```python
from build123d import *

# Parameters (mm, degrees)
F0_R     = 1.45
F1_DEPTH = 5


# Not quite as in the source:
# - ends of sketch curves that miss each other by under 0.0002 mm in the source are joined


with BuildPart() as f1:
    # F0 (on Top) → F1 (new body)
    with BuildSketch(Plane.XY):
        Polygon((-0.3545266845, 90.9670817697), (-29.9807621135, 108.0717967697), (-35.7307621135, 98.1125046262), (-37.3235262825, 82.9583658326), (-71.3455488748, 86.5342244993), (-72.5476262023, 75.0972227026), (-67.8389451324, 60.6053924919), (-100.3740420816, 50.0340986743), (-96.8203466463, 39.0969487369), (-86.6243940714, 27.7731962067), (-112.046951543, 4.8826226429), (-104.3519495698, -3.6635428501), (-90.4316983176, -9.8612380143), (-104.345925168, -41.1131032006), (-93.8401524051, -45.790574596), (-78.6025403784, -45.790574596), (-78.6025403784, -80), (-67.1025403784, -80), (-53.1822891262, -73.8023048358), (-39.2680622758, -105.0541700222), (-28.7622895129, -100.3766986268), (-18.5663369381, -89.0529460966), (6.8562205334, -111.9435196603), (14.5512225065, -103.3973541673), (19.2599035765, -88.9055239566), (51.7950005256, -99.4768177743), (55.3486959609, -88.5396678369), (53.7559317919, -73.3855290433), (87.7779543842, -69.8096703765), (86.5758770566, -58.3726685798), (78.9570710433, -45.1765094717), (108.583302492, -28.0717967697), (102.833302492, -18.1125046262), (90.5058154087, -9.1560609968), (110.6136111506, 18.5199455228), (101.3099157153, 25.2794759242), (86.4052820705, 28.4475536047), (93.5178215482, 61.9094209861), (82.2691241397, 64.3004054305), (67.364490495, 61.13232775), (60.2519510173, 94.5941951314), (49.0032536089, 92.203210687), (36.6757665257, 83.2467670575), (16.5679707838, 110.9227735772), (7.2642753485, 104.1632431758), align=None)
        with Locations((-73.1025403784, -73)):
            Circle(F0_R, mode=Mode.SUBTRACT)
        with Locations((-73.1025403784, -57)):
            Circle(F0_R, mode=Mode.SUBTRACT)
        with Locations((-37.0907187603, -96.4223002818)):
            Circle(F0_R, mode=Mode.SUBTRACT)
        with Locations((-6.5558921176, -92.4662191739)):
            Circle(F0_R, mode=Mode.SUBTRACT)
        with Locations((-43.5985050495, -81.8055729595)):
            Circle(F0_R, mode=Mode.SUBTRACT)
        with Locations((-96.4742686494, -36.9553365341)):
            Circle(F0_R, mode=Mode.SUBTRACT)
        with Locations((-89.9664823602, -22.3386092118)):
            Circle(F0_R, mode=Mode.SUBTRACT)
        with Locations((5.33442509, -103.1723088757)):
            Circle(F0_R, mode=Mode.SUBTRACT)
        with Locations((31.6202941199, -87.138616064)):
            Circle(F0_R, mode=Mode.SUBTRACT)
        with Locations((46.8371983806, -92.082887974)):
            Circle(F0_R, mode=Mode.SUBTRACT)
        with Locations((64.3290442427, -66.7439546071)):
            Circle(F0_R, mode=Mode.SUBTRACT)
        with Locations((80.2413945686, -65.0714991949)):
            Circle(F0_R, mode=Mode.SUBTRACT)
        with Locations((85.9147182049, -34.8086570489)):
            Circle(F0_R, mode=Mode.SUBTRACT)
        with Locations((99.7711246655, -26.8086570489)):
            Circle(F0_R, mode=Mode.SUBTRACT)
        with Locations((-103.1647194297, 5.4792403473)):
            Circle(F0_R, mode=Mode.SUBTRACT)
        with Locations((-91.274402222, 16.185330049)):
            Circle(F0_R, mode=Mode.SUBTRACT)
        with Locations((-92.0170529985, 46.9664067953)):
            Circle(F0_R, mode=Mode.SUBTRACT)
        with Locations((-76.8001487377, 51.9106787053)):
            Circle(F0_R, mode=Mode.SUBTRACT)
        with Locations((-64.9588021552, 80.3326548319)):
            Circle(F0_R, mode=Mode.SUBTRACT)
        with Locations((-49.0464518293, 78.6601994197)):
            Circle(F0_R, mode=Mode.SUBTRACT)
        with Locations((-12.8121778265, 91.8086570489)):
            Circle(F0_R, mode=Mode.SUBTRACT)
        with Locations((-26.668584287, 99.8086570489)):
            Circle(F0_R, mode=Mode.SUBTRACT)
        with Locations((92.6449568788, 3.1453735398)):
            Circle(F0_R, mode=Mode.SUBTRACT)
        with Locations((102.0495209155, 16.0896454498)):
            Circle(F0_R, mode=Mode.SUBTRACT)
        with Locations((83.3560408553, 40.5555404687)):
            Circle(F0_R, mode=Mode.SUBTRACT)
        with Locations((25.6374381175, 89.0825638189)):
            Circle(F0_R, mode=Mode.SUBTRACT)
        with Locations((16.2328740808, 102.0268357289)):
            Circle(F0_R, mode=Mode.SUBTRACT)
        with Locations((59.6541081021, 70.953286015)):
            Circle(F0_R, mode=Mode.SUBTRACT)
        with Locations((86.6826279084, 56.2059020804)):
            Circle(F0_R, mode=Mode.SUBTRACT)
        with Locations((56.327521049, 86.6036476267)):
            Circle(F0_R, mode=Mode.SUBTRACT)
    extrude(amount=F1_DEPTH)


solid = f1.part
```
Input: part model. Units: mm. Frame: model coordinates. A direction names the side the tool comes from. Give positions to 0.01 mm unless a question says otherwise; leave off trailing zeros. Order: outer loops, then holes, each group sorted by start corner. A loop starts at its lowest first (then second) coordinate and runs counter-clockwise, first axis right, second up. Notation, with made-up numbers: (76, -9) - (125, -9) arc R13 ccw to (125, 0) - close; hole circle Ø5 at (75.25, 9.25). An arc over 180 degrees is marked (long way). One line per item, written item: value.
1. Line query: probe 1 along X at (y, z) = (98.5, 0.2); probe 2 along Y at (x, z) = (71, 2.4); probe 3 along Y at (x, z) = (-6, 4.75). Output: solid intervals per line, ascending.
Determined:
probe 1: -35.51 to -27.29, -26.04 to -13.4, 3.99 to 25.59
probe 2: -71.57 to 61.91
probe 3: -100.37 to -93.81, -91.13 to 94.23
2. Cut plane C-C, the plane x = 73.5. Output: boundary loops of the cut face in (y, z), and give its area (3 significant figures).
Determined:
outline: (-71.31, 0) - (62.44, 0) - (62.44, 5) - (-71.31, 5) - close
area: 669 mm2
3. Draft query along X for faces 1 (the face through (105.749, -23.162, 2.465)), 2 (the face through (-73, -80, 2)), 3 (the face through (-98.62, 44.64, 2.46)), 4 (the face through (-46.323, -89.209, 2.465)). Return one class per face: released by +X, released by -X, zero draft, split by the parting line, or undercut.
Determined:
face 1: released by +X
face 2: zero draft
face 3: released by -X
face 4: undercut
4. Cut plane A-A, the plane z = 2.45. Give the number of separate pieces and of enclosed holes in the cut face, and give its area (3 significant figures).
Determined:
separate pieces: 1
enclosed holes: 30
area: 32,100 mm2
5. Reachability of faces 5 (the face through (93.563, -36.744, 2.465)), 6 (the face through (-34.09, -102.75, 2.46)), 7 (the face through (42.93, 87.79, 2.46)), 8 (the face through (-70.226, 67.953, 2.465)) from +Z, -Z, +X, -X, +Y, -Y: full face, straight path, thin tool, end or side. Return the list, or none.
Determined:
face 5: +Z, -Z, +X
face 6: +Z, -Z, -Y
face 7: +Z, -Z, +Y
face 8: +Z, -Z, -X
6. Pin query (flat end, axial travel): pin 1 Ø3.5 at (x, y) = (-6.56, -92.47) entering from +Z; pin 2 Ø2 at (y, z) = (-83.5, 3.5) entering from -X; pin 3 Ø3 at (x, z) = (75.5, 2.5) entering from +Y; pin 4 Ø1 at (y, z) = (22, 4.5) entering from +X. Return the tip coordinate at first contact, or that it passes through.
Determined:
pin 1: z = 5
pin 2: x = -49.31
pin 3: y = 63.18
pin 4: x = 106.51
7. Cut plane B-B, the plane y = 36.5. Output: boundary loops of the cut face in (x, z).
Determined:
outline: (-94.48, 0) - (88.12, 0) - (88.12, 5) - (-94.48, 5) - close
